CAD build for the part. Positions are in the model's coordinates, mm. A direction names the side the tool comes from. Round coordinates to 2 decimals unless told otherwise and drop trailing zeros. Write each loop counter-clockwise with the first axis right and the second up, starting at its lowest first coordinate (ties: lowest second). Pieces come first, ordered by that corner, then holes. Notation, with made-up numbers: (-39.75, 72) - (16.25, 72) arc R19 ccw to (16.25, 91) - close; hole circle Ø2 at (41.5, 65). An arc over 180 degrees is marked (long way). Put each result on its own line as item: value. Start each with the question number.
Item 1: Cut at B-B (y = -40.5). Give the cut face in (x, z), and give its area (3 significant figures).
Item 2: Cut at A-A (x = 26.5). Give the cut face in (y, z).
Item 3: 3-axis set-ups, long thin cutter, end or side, ignore diameter. For faces 1 (the flat face through (14, -71.8, -10)), 2 (the flat face through (-16, -71, 34.538)), 3 (the flat face through (53, -71, 34.538)), 4 (the flat face through (-9.412, -35, 13)), 5 (the cylindrical face through (53.398, -6.915, 53.962)): which of +Z, -Z, +X, -X, +Y, -Y reach the whole face in a straight line?
Item 4: Cut at C-C (z = 57.5). Give the cut face in (x, y), and give its area (3 significant figures).
Item 5: Drill centre lines: line 1 (Z direction, x = 20.5, y = -0.5); line 2 (X direction, y = -59, z = 3.5); line 3 (Y direction, x = 37, z = -13). Where is each one in solid material? Low to high. Write a range as from..to.
Item 6: Mould opens along Z. For faces 6 (the cylindrical face through (-12.73, -71.68, 53.96)), 7 (the flat face through (17, -35, 23.926)), 8 (the flat face through (19, -75, -15.017)), 9 (the flat face through (19, -35, 34.538)) say: released by +Z, released by -Z, zero draft, split by the parting line, or undercut.
Item 7: Cut at D-D (z = 28.5). Give the cut face in (x, y).
Item 8: Pin check, flat tips, straight feed: pin 1 Ø16 at (x, y) = (28.5, -23.5) entering from -Z; pin 2 Ø8 at (x, y) = (11.5, -19) entering from +Z; pin 3 Ø4 at (x, z) = (33, 3.5) entering from +Y. Stop position of each tip, or through.
```python
from build123d import *

# Parameters (mm, degrees)
F1_DEPTH  = 71.8
F2_R      = 5
F3_DEPTH  = 39.4
F4_W      = 9
F4_H      = 10
F5_DEPTH  = 7
F6_W      = 9
F6_H      = 10
F7_DEPTH  = 7
F5_FACE_W = 7
F5_FACE_H = 10
F8_DEPTH  = 62
F7_FACE_W = 7
F7_FACE_H = 10
F9_DEPTH  = 62


with BuildPart() as f1:
    # F0 (on Front) → F1 (new body)
    with BuildSketch(Plane.XZ):
        Polygon((43.408085, -3.087412), (43.408085, -44.812847), (53.779151, -44.57166), (53.779151, 34.537837), (-16.647598, 34.537837), (-16.647598, 23.925588), (-9.411974, 23.925588), (43.408085, 23.925588), (43.408085, 3.183464), align=None)
        Polygon((-16.647598, -3.087412), (43.408085, -3.087412), (43.408085, 3.183464), (-9.411974, 3.183464), (-9.411974, 23.925588), (-16.647598, 23.925588), align=None)
    extrude(amount=F1_DEPTH)

    # F2 (on face) → F3 (join)
    with BuildSketch(Plane.XY.offset(34.537837)):
        with BuildLine():
            ThreePointArc((-16.647598, -66.8), (-11.647598, -71.8), (-6.647598, -66.8))
            ThreePointArc((-6.647598, -66.8), (-11.647598, -61.8), (-16.647598, -66.8))
        make_face()
        with Locations((48.779151, -66.8)):
            Circle(F2_R)
        with Locations((48.779151, -5)):
            Circle(F2_R)
        with BuildLine():
            ThreePointArc((-16.647598, -5), (-11.647598, -10), (-6.647598, -5))
            ThreePointArc((-6.647598, -5), (-11.647598, 0), (-16.647598, -5))
        make_face()
    extrude(amount=F3_DEPTH)

    # F4 (on face) → F5 (join)
    with BuildSketch(Plane.XZ.offset(71.8)):
        with Locations((49.279151, -10.016912)):
            Rectangle(F4_W, F4_H)
    extrude(amount=F5_DEPTH)

    # F6 (on face) → F7 (join)
    with BuildSketch(Plane(origin=(0, 0, 0), x_dir=(-1, 0, 0), z_dir=(0, 1, 0))):
        with Locations((-49.279151, -10.016912)):
            Rectangle(F6_W, F6_H)
    extrude(amount=F7_DEPTH)

    # F5_face (on face) → F8 (join)
    with BuildSketch(Plane(origin=(44.779151, -75.3, -10.016912), x_dir=(0, -1, 0), z_dir=(-1, 0, 0))):
        Rectangle(F5_FACE_W, F5_FACE_H)
    extrude(amount=F8_DEPTH)

    # F7_face (on face) → F9 (join)
    with BuildSketch(Plane(origin=(44.779151, 3.5, -10.016912), x_dir=(0, -1, 0), z_dir=(-1, 0, 0))):
        Rectangle(F7_FACE_W, F7_FACE_H)
    extrude(amount=F9_DEPTH)


solid = f1.part
```
Output values:
1. outline: (-16.65, -3.09) - (43.41, -3.09) - (43.41, -44.81) - (53.78, -44.57) - (53.78, 34.54) - (-16.65, 34.54) - close; hole (-9.41, 3.18) - (43.41, 3.18) - (43.41, 23.93) - (-9.41, 23.93) - close
1. area: 1,990 mm2
2. outline: (-78.8, -15.02) - (-71.8, -15.02) - (-71.8, -5.02) - (-78.8, -5.02) - close; (-71.8, -3.09) - (0, -3.09) - (0, 3.18) - (-71.8, 3.18) - close; (-71.8, 23.93) - (0, 23.93) - (0, 34.54) - (-71.8, 34.54) - close; (0, -15.02) - (7, -15.02) - (7, -5.02) - (0, -5.02) - close
3. face 1: -Z, -X
3. face 2: +Z, -X, -Y
3. face 3: +Z, +X, -Y
3. face 4: +Y, -Y
3. face 5: +Z
4. outline: circle Ø10 at (-11.65, -66.8); circle Ø10 at (-11.65, -5); circle Ø10 at (48.78, -66.8); circle Ø10 at (48.78, -5)
4. area: 314 mm2
5. line 1: -3.09..3.18, 23.93..34.54
5. line 2: -16.65..-9.41, 43.41..53.78
5. line 3: -78.8..-71.8, 0..7
6. face 6: zero draft
6. face 7: undercut
6. face 8: released by -Z
6. face 9: released by +Z
7. outline: (-16.65, -71.8) - (53.78, -71.8) - (53.78, 0) - (-16.65, 0) - close
8. pin 1: z = -3.09
8. pin 2: z = 34.54
8. pin 3: y = 0
